from build123d import *

# Parameters (mm, degrees)
CROQUIS1_W                     = 127
CROQUIS1_H                     = 125
BRIDA_BASE1_DEPTH              = 3.175
CROQUIS11_R                    = 10.05
CORTAR_EXTRUIR3_DEPTH          = 10
TALADRO_DE_MARGEN_PARA_M51_D   = 5.2
TALADRO_DE_MARGEN_PARA_M52_D   = 5.2
CROQUIS16_R                    = 5
CORTAR_EXTRUIR4_DEPTH          = 127.234229213
CROQUIS17_R                    = 14
CROQUIS17_R_2                  = 4.75
CORTAR_EXTRUIR5_DEPTH          = 10
TALADRO_DE_MARGEN_PARA_M3_51_D = 3.9
REDONDEO1_R                    = 40


# Sheet-metal steps are written as plain solids
with BuildPart() as part:
    # Croquis1 → Brida base1 (new body)
    with BuildSketch(Plane(origin=(0, 0, 0), x_dir=(1, 0, 0), z_dir=(0, 1, 0))):
        with Locations((-41.5, 7.5)):
            Rectangle(CROQUIS1_W, CROQUIS1_H)
    extrude(amount=-BRIDA_BASE1_DEPTH)

    # Croquis11 → Cortar-Extruir3 (cut)
    with BuildSketch(Plane(origin=(0, 0, 0), x_dir=(1, 0, 0), z_dir=(0, 1, 0))):
        with Locations(Location((0, 0, 0), (0, 0, 270))):
            Circle(CROQUIS11_R)
    extrude(amount=-CORTAR_EXTRUIR3_DEPTH, mode=Mode.SUBTRACT)

    # Taladro de margen para M51 (through all)
    with Locations(Plane(origin=(0, 0, 0), x_dir=(1, 0, 0), z_dir=(0, 1, 0))):
        with Locations((17, 17), (-17, 17), (-17, -17), (17, -17)):
            Hole(TALADRO_DE_MARGEN_PARA_M51_D / 2)

    # Taladro de margen para M52 (through all)
    with Locations(Plane(origin=(0, 0, 0), x_dir=(1, 0, 0), z_dir=(0, 1, 0))):
        with Locations((-37.578650523, 34.25587131), (-37.434837835, -12.743908668), (-84.434617812, -12.887721356), (-84.578430501, 34.112058621), (-61.006634168, 10.684074977)):
            Hole(TALADRO_DE_MARGEN_PARA_M52_D / 2)

    # Croquis16 → Cortar-Extruir4 (cut, through all)
    with BuildSketch(Plane(origin=(0, 0, 0), x_dir=(1, 0, 0), z_dir=(0, 1, 0))):
        with Locations(Location((-61.006634168, 10.684074977, 0), (0, 0, 270))):
            Circle(CROQUIS16_R)
    extrude(amount=-CORTAR_EXTRUIR4_DEPTH, mode=Mode.SUBTRACT)

    # Croquis17 → Cortar-Extruir5 (cut)
    with BuildSketch(Plane(origin=(0, 0, 0), x_dir=(1, 0, 0), z_dir=(0, 1, 0))):
        with Locations(Location((-32.425079896, -39.098203149, 0), (0, 0, 270))):
            Circle(CROQUIS17_R)
        with Locations(Location((2, 50, 0), (0, 0, 270))):
            Circle(CROQUIS17_R_2)
    extrude(amount=-CORTAR_EXTRUIR5_DEPTH, mode=Mode.SUBTRACT)

    # Taladro de margen para M3.51 (through all)
    with Locations(Plane(origin=(-235.296017462, -6.288, -137.590485756), x_dir=(-0.5911403395410236, 0, 0.806568719308729), z_dir=(0, -1, 0))):
        with Locations((46.983235392, -222.472189169), (42.30898943, -237.296741799), (-48.324723402, -208.719537692), (-43.650477439, -193.894985062)):
            Hole(TALADRO_DE_MARGEN_PARA_M3_51_D / 2)

    # Redondeo1
    redondeo1_edges = [part.edges().sort_by_distance(p)[0] for p in [
        (22, -1.5875, 55),
        (-105, -1.5875, 55),
        (-105, -1.5875, -70),
        (22, -1.5875, -70),
    ]]
    fillet(redondeo1_edges, radius=REDONDEO1_R)


solid = part.part
Geometry check sheet. Reference: the model listing, model coordinates, mm. Round coordinates to 2 decimals unless told otherwise and drop trailing zeros. Loops run counter-clockwise (first coordinate to the right, second up) from the corner with the lowest first, then second, coordinate; pieces in that order, holes last. Notation, with made-up numbers: (25.25, -37) - (81.25, -37) arc R11 ccw to (81.25, -24) - close; hole circle Ø11 at (84, -40). An arc over 180 degrees is marked (long way). Answer as CSV lines item,"result".
(1) Depth check by flat-ended pin: pin 1 Ø3 at (x, z) = (-37.43, 12.74) entering from -Y; pin 2 Ø7 at (x, z) = (17, -17) entering from +Y. Enter the tip coordinate at first touch or a pass-through.
Output values:
pin 1,"passes through"
pin 2,"stops at y = 0"
(2) Cross-section at C-C, the plane z = 17. Enter the section's corners in (x, y) (3 decimals), and give its area (3 significant figures).
Output values:
outline,"(-104.95, -3.175) - (-19.6, -3.175) - (-19.6, 0) - (-104.95, 0) - close; (-14.4, -3.175) - (14.4, -3.175) - (14.4, 0) - (-14.4, 0) - close; (19.6, -3.175) - (21.95, -3.175) - (21.95, 0) - (19.6, 0) - close"
area,"370 mm²"
(3) Cross-section at A-A, the plane z = 0. Enter the section's corners in (x, y) (3 decimals).
Output values:
outline,"(-105, -3.175) - (-10.05, -3.175) - (-10.05, 0) - (-105, 0) - close; (10.05, -3.175) - (22, -3.175) - (22, 0) - (10.05, 0) - close"
(4) Cross-section at D-D, the plane y = -2.35. Give the number of separate pieces and of enclosed holes in the cut face, and give its area (3 significant figures).
Output values:
separate pieces,"1"
enclosed holes,"16"
area,"13,200 mm²"
(5) Release check for a two-part mould opening along X. For faces 1 (the face through (-84.85, -1.57, 33.34)), 2 (the face through (9.972, -1.61, -58.594)), 3 (the face through (-42, -2, -70)) record: released by +X, released by -X, zero draft, split by the parting line, or undercut.
Output values:
face 1,"undercut"
face 2,"released by +X"
face 3,"zero draft"
(6) Cross-section at B-B, the plane x = 17. Enter the section's corners in (y, z) (3 decimals), and give its area (3 significant figures).
Output values:
outline,"(-3.175, -49.365) - (0, -49.365) - (0, -19.6) - (-3.175, -19.6) - close; (-3.175, -14.4) - (0, -14.4) - (0, 14.4) - (-3.175, 14.4) - close; (-3.175, 19.6) - (0, 19.6) - (0, 34.365) - (-3.175, 34.365) - close"
area,"233 mm²"
(7) Material ranges on line 1 along Z through (x, y) = (17, -2.2); line 2 along Z through (x, y) = (-17, -0.85); line 3 along Z through (x, y) = (-60.5, -2.75), recorded low to high.
Output values:
line 1,"z = -49.36 to -19.6, -14.4 to 14.4, 19.6 to 34.36"
line 2,"z = -69.99 to -19.6, -14.4 to 14.4, 19.6 to 54.99"
line 3,"z = -70 to -15.66, -5.71 to 55"
